from build123d import *

# Parameters (mm, degrees)
BOSS_EXTRUDE1_DEPTH = 50
CUT_EXTRUDE1_DEPTH  = 110.24284873619861
FILLET1_R           = 10
HOLE1_D             = 10
HOLE2_D             = 10


with BuildPart() as part:
    # Sketch1 → Boss-Extrude1 (new body)
    with BuildSketch(Plane.XY):
        Polygon((-10, 0), (10, 3.67e-15), (9.999999999999991, 50.00000000000001), (-52.35382907247969, 85.99999999999983), (-62.35382907247966, 68.67949192431102), (-10.000000000000009, 38.45299461620743), align=None)
    extrude(amount=BOSS_EXTRUDE1_DEPTH)

    # Sketch2 → Cut-Extrude1 (cut, through all)
    with BuildSketch(Plane(origin=(24.150635094610877, 41.83012701892233, 0), x_dir=(0.86602540378444, -0.4999999999999976, 0), z_dir=(0.4999999999999976, 0.86602540378444, 0))):
        with BuildLine():
            Line((-72.33974596215559, -50), (-88.33974596215548, -50))
            Line((-88.33974596215548, -50), (-88.33974596215548, 0))
            Line((-88.33974596215548, 0), (-72.33974596215559, -6.94e-15))
            ThreePointArc((-72.33974596215559, -6.94e-15), (-67.33974596215559, -5.000000000000008), (-72.33974596215559, -10.000000000000009))
            ThreePointArc((-72.33974596215559, -10.000000000000009), (-87.33974596215559, -25.000000000000007), (-72.33974596215559, -40.000000000000014))
            ThreePointArc((-72.33974596215559, -40.000000000000014), (-67.33974596215559, -45.000000000000014), (-72.33974596215559, -50))
        make_face()
    extrude(amount=-CUT_EXTRUDE1_DEPTH, mode=Mode.SUBTRACT)

    # Fillet1
    fillet1_edges = [part.edges().sort_by_distance(p)[0] for p in [
        (-43.49742261192873, 69.33974596215553, 7.47e-15),
        (-43.49742261192873, 69.33974596215553, 50),
    ]]
    fillet(fillet1_edges, radius=FILLET1_R - 0.0001)  # a hair under: the kernel refuses the full size

    # Hole1 (through all)
    with Locations(Plane(origin=(24.150635094610877, 41.83012701892233, 0), x_dir=(0.86602540378444, -0.4999999999999976, 0), z_dir=(0.4999999999999976, 0.86602540378444, 0))):
        with Locations((-72.339745962, -25)):
            Hole(HOLE1_D / 2)

    # Hole2 (through all)
    with Locations(Plane(origin=(10, 1.73e-15, 0), x_dir=(0, 0, -1), z_dir=(1, 1.7e-16, 0))):
        with Locations((-37.675212833, 17.399574334), (-11.057265884, 17.399574334)):
            Hole(HOLE2_D / 2)


solid = part.part
Work out the finished part from the listing and answer in its coordinate system (mm). A direction names the side the tool comes from. Give positions to 0.01 mm unless a question says otherwise; leave off trailing zeros. Order: outer loops, then holes, each group sorted by start corner. A loop starts at its lowest first (then second) coordinate and runs counter-clockwise, first axis right, second up. Notation, with made-up numbers: (67.5, 56.25) - (123.5, 56.25) arc R15 ccw to (123.5, 70.25) - close; hole circle Ø4 at (7, 58.5). An arc over 180 degrees is marked (long way). Answer as CSV lines item,"result". Start each with the question number.
Q1. The part is cut by section C-C (x = -4). Write down the section's boundary in (y, z), then the cut area to 3 significant figures.
Q2. The part is cut by section A-A (z = 14.5). Write down the section's boundary in (x, y).
Q3. Given pin 1 Ø4 at (x, y) = (-30, 69) entering from -Z; pin 2 Ø1 at (y, z) = (18.5, 27) entering from -X; pin 3 Ø3 at (x, z) = (-37.5, 26) entering from +Y; pin 4 Ø6 at (y, z) = (17.4, 37.68) entering from -X, each flat-ended and moving along its own axis, determine where each tip first touches the part or whether it passes through.
Q4. Find the intervals of material crossed by L1, parallel to X at y = 8, z = 45; L2, parallel to Y at x = -4, z = 41; L3, parallel to Y at x = 5.5, z = 36, in increasing order. Write a range as [from, to].
Q5. The part is cut by section B-B (y = 19.5). Write down the section's boundary in (x, z).
Q6. The part is cut by section D-D (z = 31). Write down the section's boundary in (x, y).
Q7. For faces 1 (the face through (-10, 19, 25)), 2 (the face through (-45.566, 70.372, 29.436)), determine the directions among +Z, -Z, +X, -X, +Y, -Y from which every point of the face is accessible in a straight line to the end or side of a thin tool.
Q8. The mould has two halves that part along Z. Classify faces 3 (the face through (-8, 36, 0)), 4 (the face through (-8, 36, 50)), 5 (the face through (-0.14, 18.901, 15.826)), 6 (the face through (-13.482, 63.557, 24.65)): +Z half, -Z half, draft (parallel to the pull), parting line (faces both ways), or undercut.
Check result:
1,outline,"(0, 0) - (58.08, 0) - (58.08, 50) - (0, 50) - close; hole circle Ø10 at (17.4, 11.06); hole circle Ø10 at (17.4, 37.68)"
1,area,"2,750 mm²"
2,outline,"(-57.77, 66.04) - (-10, 38.45) - (-10, 21.03) - (10, 21.03) - (10, 50) - (-47.77, 83.36) - close; (-10, 0) - (10, 0) - (10, 13.77) - (-10, 13.77) - close"
3,pin 1,"stops at z = 0"
3,pin 2,"stops at x = -10"
3,pin 3,"stops at y = 72.64"
3,pin 4,"passes through"
4,L1,"x = [-10, 10]"
4,L2,"y = [0, 13.67], [21.13, 58.08]"
4,L3,"y = [0, 12.69], [22.11, 52.6]"
5,outline,"(-10, 0) - (10, 0) - (10, 6.52) - (-10, 6.52) - close; (-10, 15.59) - (10, 15.59) - (10, 33.14) - (-10, 33.14) - close; (-10, 42.21) - (10, 42.21) - (10, 50) - (-10, 50) - close"
6,outline,"(-60.4, 67.55) - (-10, 38.45) - (-10, 0) - (10, 0) - (10, 50) - (-50.4, 84.87) - close"
7,face 1,"+Z, -Z, -X, -Y"
7,face 2,"none"
8,face 3,"-Z half"
8,face 4,"+Z half"
8,face 5,"undercut"
8,face 6,"draft"
